Build history of the part. All positions in model axes, mm. Round coordinates to 2 decimals unless told otherwise and drop trailing zeros. Loops run counter-clockwise (first coordinate to the right, second up) from the corner with the lowest first, then second, coordinate; pieces in that order, holes last. Notation, with made-up numbers: (43, 38.25) -> (77, 38.25) arc R19 ccw to (77, 46.25) -> close; hole circle Ø3 at (-33, -10.5). An arc over 180 degrees is marked (long way). Put each result on its own line as item: value. Start each with the question number.
Item 1: Pull direction X, two halves, no side cores. Call faces 1 (the flat face through (0, -81, 0.2)), 2 (the cylindrical face through (-30.75, -80.96, 10.02)), 3 (the flat face through (31.92, -81, 68)): +X half, -X half, draft (parallel to the pull), parting line (faces both ways), or undercut.
Item 2: Flat gauge pin, fed straight in: pin 1 Ø4.5 at (x, z) = (-29.68, 9.2) entering from -Y. Where does the tip first touch, or does it go through?
Item 3: Cut at A-A, the plane z = 9.2. List the corners of the cut face in (x, y).
Item 4: Drill centre lines: probe 1 along X at (y, z) = (-82.4, 9.2); probe 2 along X at (y, z) = (-83.3, 128.5). Where is each one in solid material? Low to high. Write a range as [from, to].
Autodesk Inventor part; units mm, degrees
ref_plane "YZ Plane" through (0, 0, 0) normal (1, 0, 0) x (0, 1, 0)
ref_plane "XZ Plane" through (0, 0, 0) normal (0, 1, 0) x (-1, 0, 0)
ref_plane "XY Plane" through (0, 0, 0) normal (0, 0, 1) x (1, 0, 0)
sketch "스케치1" plane through (0, 0, 0.2) normal (0, 0, 1) x (1, 0, 0)
  circle A0 centre (-22.9203, -41.3997) radius 1.35
  circle A1 centre (-22.9203, 35.0003) radius 1.35
  line L0 (-31.9205, -84) -> (-31.9205, 78)
  line L1 (31.9205, -84) -> (-31.9205, -84)
  line L2 (31.9205, 78) -> (31.9205, -84)
  line L3 (-31.9205, 78) -> (31.9205, 78)
  circle A2 centre (-22.9203, -75) radius 1.45
  circle A3 centre (-22.9203, 69) radius 1.45
  line L4 (-31.9205, -84) -> (31.9205, -84)
  line L5 (31.9205, -84) -> (31.9205, -78)
  line L6 (31.9205, -78) -> (-31.9205, -78)
  line L7 (-31.9205, -78) -> (-31.9205, -84)
  point P0 (0, 0)
  point P1 (-31.9205, -78)
extrude "돌출1" add sketch "스케치1" along normal blind 136.628 contours L0 L6 L2 L1
sketch "스케치4" plane through (-31.9205, -84, 0.2) normal (0, -1, 0) x (1, 0, 0)
  circle A0 centre (2.641, 9) radius 1.35
  circle A1 centre (2.641, 75.2636) radius 1.35
  point P0 (31.9205, -0.2)
extrude "돌출4" cut sketch "스케치4" against normal through all contours A1
sketch "스케치5" plane through (-31.9205, -84, 0.2) normal (0, -1, 0) x (1, 0, 0)
  circle A0 centre (2.641, 127.428) radius 1.35
  point P0 (31.9205, -0.2)
extrude "돌출5" cut sketch "스케치5" against normal up to next
sketch "스케치6" plane through (-31.9205, -78, 0.2) normal (0, 1, 0) x (1, 0, 0)
  circle A0 centre (2.241, -9) radius 1.35
  point P0 (31.9205, 0.2)
extrude "돌출6" cut sketch "스케치6" against normal up to next
properties part number "부품82" material "PMMA 플라스틱"
Reply:
1. face 1: draft
1. face 2: undercut
1. face 3: +X half
2. pin 1: stops at y = -84
3. outline: (-31.92, -84) -> (-31.03, -84) -> (-31.03, -78) -> (-31.92, -78) -> close; (-28.33, -84) -> (31.92, -84) -> (31.92, -78) -> (-28.33, -78) -> close
4. probe 1: x = [-31.92, -31.03], [-28.33, 31.92]
4. probe 2: x = [-31.92, -30.31], [-28.25, 31.92]
